from build123d import *

# Parameters (mm, degrees)
F0_R     = 5
F0_R_2   = 4
F1_DEPTH = 29
F2_SIZE  = 0.25


with BuildPart() as f1:
    # F0 (on Right) → F1 (new body)
    with BuildSketch(Plane.YZ):
        Circle(F0_R)
        Circle(F0_R_2, mode=Mode.SUBTRACT)
    extrude(amount=F1_DEPTH)

    # F2
    f2_edges = [f1.edges().sort_by_distance(p)[0] for p in [
        (29, -5, 0),
        (0, -5, 0),
        (0, -4, 0),
        (29, -4, 0),
    ]]
    chamfer(f2_edges, length=F2_SIZE)


solid = f1.part
Verification items for the finished model (mm, model axes). Coordinates: 2 decimals unless noted, no trailing zeros. Order: outer loops, then holes, each group sorted by start corner. A loop starts at its lowest first (then second) coordinate and runs counter-clockwise, first axis right, second up. Notation, with made-up numbers: M 3.25,10 L 47.25,10 A25 ccw 47.25,48 Z; hole C 82.5,-13 d2. An arc over 180 degrees is marked long. One line per item, written item: value. Start each with the question number.
Item 1: Sectioned sample at C-C (x = 26.25). Enter the section's corners in (y, z).
Item 2: Scan lines: probe 1 along Z at (x, y) = (14, 0); probe 2 along Z at (x, y) = (20.5, -3); probe 3 along Y at (x, z) = (10, 3.5). Record each from-to range of solid material in increasing order.
Item 3: Mould release check, pull along Z, two halves, no side actions. Record for faces 1 (the flat face through (29, -4, -2)), 2 (the cylindrical face through (14.3, -0.867, -3.905)), 3 (the cylindrical face through (14.3, -1.08, -4.88)): released by +Z, released by -Z, zero draft, split by the parting line, or undercut.
Item 4: Gauge pin test, flat ends, axial feed: pin 1 (1 mm diameter, centred on x = 14, z = -2, fed in from -Y); pin 2 (4 mm diameter, centred on x = 25, z = -3.5, fed in from +Y); pin 3 (6 mm diameter, centred on x = 16.5, y = -3.5, fed in from -Z). Record the tip position at first contact, or that the pin passes through.
Item 5: Sectioned sample at A-A (z = 0). Enter the section's corners in (x, y), then the cut area to 4 significant figures.
Conclusion:
1. outline: C 0,0 d10; hole C 0,0 d8
2. probe 1: z = -5 to -4, 4 to 5
2. probe 2: z = -4 to -2.65, 2.65 to 4
2. probe 3: y = -3.57 to -1.94, 1.94 to 3.57
3. face 1: zero draft
3. face 2: undercut
3. face 3: split by the parting line
4. pin 1: stops at y = -4.77
4. pin 2: stops at y = 4.77
4. pin 3: stops at z = -4.97
5. outline: M 0,-4.75 L 0.25,-5 L 28.75,-5 L 29,-4.75 L 29,-4.25 L 28.75,-4 L 0.25,-4 L 0,-4.25 Z; M 0,4.25 L 0.25,4 L 28.75,4 L 29,4.25 L 29,4.75 L 28.75,5 L 0.25,5 L 0,4.75 Z
5. area: 57.75 mm^2
